Source: CAD feature listing. Evaluate the final solid. Frame: model axes, mm. Give positions to 0.01 mm unless a question says otherwise; leave off trailing zeros. Order: outer loops, then holes, each group sorted by start corner. A loop starts at its lowest first (then second) coordinate and runs counter-clockwise, first axis right, second up. Notation, with made-up numbers: M 28.5,10 L 84.5,10 A18 ccw 84.5,31 Z; hole C 6,7 d9. An arc over 180 degrees is marked long. One line per question, with ' | ' between items. Start each with the question number.
from build123d import *

# Parameters (mm, degrees)
SKETCH_1_R      = 2.75
SKETCH_1_R_2    = 4
EXTRUDE_1_DEPTH = 3
SKETCH_2_R      = 10
SKETCH_2_R_2    = 4
EXTRUDE_2_DEPTH = 4


with BuildPart() as part:
    # 草图1 → 凸台-拉伸1 (new body)
    with BuildSketch(Plane(origin=(0, 0, 0), x_dir=(1, 0, 0), z_dir=(0, 1, 0))):
        with BuildLine():
            Line((-19.5, 3.5), (-19.5, -3.5))
            Line((-19.5, -3.5), (-3.443077457, -9.388568455))
            ThreePointArc((-3.443077457, -9.388568455), (0, -10), (3.443077457, -9.388568455))
            Line((3.443077457, -9.388568455), (19.5, -3.5))
            Line((19.5, -3.5), (19.5, 3.5))
            Line((19.5, 3.5), (3.443077457, 9.388568455))
            ThreePointArc((3.443077457, 9.388568455), (0, 10), (-3.443077457, 9.388568455))
            Line((-3.443077457, 9.388568455), (-19.5, 3.5))
        make_face()
        with Locations(Location((-16, 0, 0), (0, 0, 270))):
            Circle(SKETCH_1_R, mode=Mode.SUBTRACT)
        with Locations(Location((0, 0, 0), (0, 0, 270))):
            Circle(SKETCH_1_R_2, mode=Mode.SUBTRACT)
        with Locations(Location((16, 0, 0), (0, 0, 90))):
            Circle(SKETCH_1_R, mode=Mode.SUBTRACT)
    extrude(amount=EXTRUDE_1_DEPTH)

    # 草图2 → 凸台-拉伸2 (add)
    with BuildSketch(Plane(origin=(0, 3, 0), x_dir=(1, 0, 0), z_dir=(0, 1, 0))):
        with Locations(Location((0, 0, 0), (0, 0, 110.139543726))):
            Circle(SKETCH_2_R)
        with Locations(Location((0, 0, 0), (0, 0, 270))):
            Circle(SKETCH_2_R_2, mode=Mode.SUBTRACT)
    extrude(amount=EXTRUDE_2_DEPTH)


solid = part.part
Item 1: Cut plane D-D on y = 4. Return the cut outline in (x, z), and give its area (3 significant figures).
Item 2: Cut plane A-A on x = 0. Return the cut outline in (y, z).
Item 3: Mould query, pull axis Z, two halves, no side actions, for faces 1 (the cylindrical face through (-3.905, 3.451, -0.867)), 2 (the flat face through (-11.584, 1.479, 6.403)), 3 (the flat face through (-11.359, 1.479, -6.486)). Classes: pulls with the +Z half, pulls with the -Z half, needs draft (parallel to the pull), parting line crosses it, or undercut.
Item 4: Pin query (flat end, axial travel): pin 1 Ø1 at (y, z) = (5, -0.5) entering from -X; pin 2 Ø10 at (x, z) = (-14, 8) entering from -Y; pin 3 Ø7 at (x, z) = (16, 0) entering from +Y; pin 4 Ø2 at (x, y) = (7, 6) entering from -Z. Return the tip coordinate at first contact, or that it passes through.
Item 5: Cut plane C-C on y = 2.25. Return the cut outline in (x, z).
Item 6: Line query: line 1 (X direction, y = 1.85, z = 0); line 2 (X direction, y = 1.25, z = -1.5); line 3 (Y direction, x = -15.5, z = -4). Output: solid intervals per line, ascending.
Item 7: Cut plane B-B on z = 0. Return the cut outline in (x, y), and give its area (3 significant figures).
Results are:
1) outline: C 0,0 d20; hole C 0,0 d8 | area: 264 mm2
2) outline: M 0,-10 L 7,-10 L 7,-4 L 0,-4 Z; M 0,4 L 7,4 L 7,10 L 0,10 Z
3) face 1: undercut | face 2: pulls with the +Z half | face 3: pulls with the -Z half
4) pin 1: stops at x = -10 | pin 2: stops at y = 0 | pin 3: stops at y = 3 | pin 4: stops at z = -8
5) outline: M -19.5,-3.5 L -3.44,-9.39 A10 ccw 3.44,-9.39 L 19.5,-3.5 L 19.5,3.5 L 3.44,9.39 A10 ccw -3.44,9.39 L -19.5,3.5 Z; hole C -16,0 d5.5; hole C 0,0 d8; hole C 16,0 d5.5
6) line 1: x = -19.5 to -18.75, -13.25 to -4, 4 to 13.25, 18.75 to 19.5 | line 2: x = -19.5 to -18.3, -13.7 to -3.71, 3.71 to 13.7, 18.3 to 19.5 | line 3: y = 0 to 3
7) outline: M -19.5,0 L -18.75,0 L -18.75,3 L -19.5,3 Z; M -13.25,0 L -4,0 L -4,7 L -10,7 L -10,3 L -13.25,3 Z; M 4,0 L 13.25,0 L 13.25,3 L 10,3 L 10,7 L 4,7 Z; M 18.75,0 L 19.5,0 L 19.5,3 L 18.75,3 Z | area: 108 mm2
